Geometry: see drawing. Coordinates: mm, zero at the bounding-box minimum. A direction names the side the tool comes from. Give positions to 0.01 mm unless a question says otherwise; leave off trailing zeros. Write each loop counter-clockwise with the first axis right and the second up, starting at its lowest first coordinate (ties: lowest second). Pieces come first, ordered by that corner, then holes. Notation, with made-up numbers: M -35,-16.5 L 4,-16.5 A21 ccw 4,6.5 Z; hole C -27.75,11 d4. An arc over 180 degrees is marked long. Use a Markdown table: item, result. Add a question column.
(1) Cut plane D-D (z = 40). Output: boundary loops of the cut face in (x, y).
(2) Reachability of the marked faces 1, 2 and 3 from +Z, -Z, +X, -X, +Y, -Y: full face, straight path, thin tool, end or side. Return the list, or none.
(3) Cut plane C-C (x = 19). Output: boundary loops of the cut face in (y, z), plus the area to 3 significant figures.
(4) Cut plane B-B (z = 65). Output: boundary loops of the cut face in (x, y).
(5) Cut plane A-A (y = 60). Output: boundary loops of the cut face in (x, z).
(6) Pin query (flat end, axial travel): pin 1 Ø5.5 at (y, z) = (60, 15) entering from +X; pin 2 Ø4 at (x, y) = (42.5, 45.5) entering from -Z; pin 3 Ø2 at (y, z) = (47.5, 55) entering from +X; pin 4 Ø8 at (y, z) = (10, 15) entering from -X. Return the tip coordinate at first contact, or that it passes through.
(7) Material intervals for L1, parallel to Z at x = 18.25, y = 10; L2, parallel to Y at x = 21, z = 15; L3, parallel to X at y = 6, z = 42, sorted ascending.
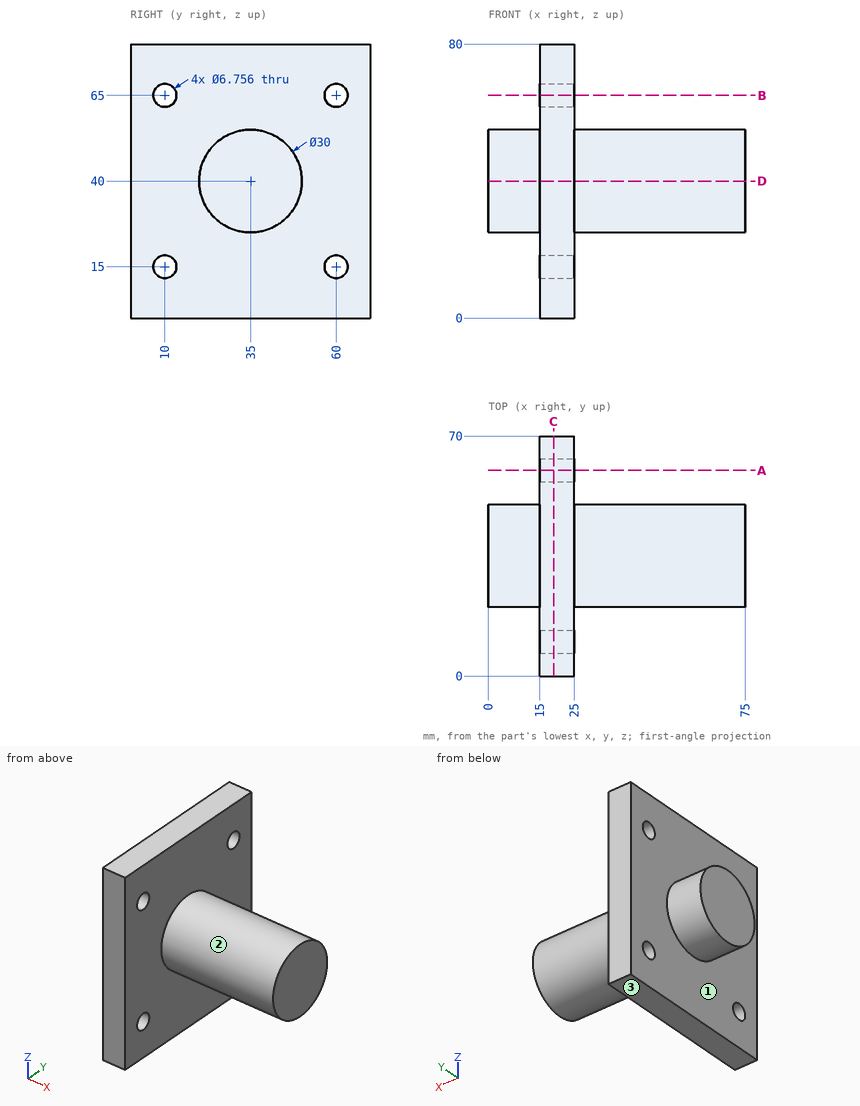
Answer list:
| question | item | result |
|---|---|---|
| 1 | outline | M 0,20 L 15,20 L 15,0 L 25,0 L 25,20 L 75,20 L 75,50 L 25,50 L 25,70 L 15,70 L 15,50 L 0,50 Z |
| 2 | face 1 | -X |
| 2 | face 2 | +X |
| 2 | face 3 | -Z, +X, -X, +Y, -Y |
| 3 | outline | M 0,0 L 70,0 L 70,80 L 0,80 Z; hole C 10,15 d6.76; hole C 10,65 d6.76; hole C 60,15 d6.76; hole C 60,65 d6.76 |
| 3 | area | 5,460 mm² |
| 4 | outline | M 15,0 L 25,0 L 25,6.62 L 15,6.62 Z; M 15,13.38 L 25,13.38 L 25,56.62 L 15,56.62 Z; M 15,63.38 L 25,63.38 L 25,70 L 15,70 Z |
| 5 | outline | M 15,0 L 25,0 L 25,11.62 L 15,11.62 Z; M 15,18.38 L 25,18.38 L 25,61.62 L 15,61.62 Z; M 15,68.38 L 25,68.38 L 25,80 L 15,80 Z |
| 6 | pin 1 | through |
| 6 | pin 2 | z = 27.64 |
| 6 | pin 3 | x = 25 |
| 6 | pin 4 | x = 15 |
| 7 | L1 | 0 to 11.62, 18.38 to 61.62, 68.38 to 80 |
| 7 | L2 | 0 to 6.62, 13.38 to 56.62, 63.38 to 70 |
| 7 | L3 | 15 to 25 |
